For this review, take the finished solid that the model builds, in its own axes (mm). A direction names the side the tool comes from. Give positions to 0.01 mm unless a question says otherwise; leave off trailing zeros. Write each loop counter-clockwise with the first axis right and the second up, starting at its lowest first coordinate (ties: lowest second). Pieces come first, ordered by that corner, then holes.
from build123d import *

# Parameters (mm, degrees)
CHAMFER1_SIZE = 0.254
CHAMFER2_SIZE = 0.127


with BuildPart() as part:
    # Sketch1 → Revolve1 (revolve)
    with BuildSketch(Plane(origin=(0, 0, 0), x_dir=(0, 0, -1), z_dir=(1, 0, 0)), mode=Mode.PRIVATE) as revolve1_sk:
        Polygon((0, 6.35), (25.4, 6.35), (25.4, 4.6736), (15.24, 4.6736), (15.24, 3.96875), (0, 3.96875), align=None)
    revolve(revolve1_sk.sketch.rotate(Axis((0, 0, 0), (0, 0, -1)), 90), axis=Axis((0, 0, 0), (0, 0, -1)))

    # Chamfer1
    chamfer1_edges = [part.edges().sort_by_distance(p)[0] for p in [
        (-3.96875, 0, 0),
        (-4.6736, 0, -25.4),
        (-6.35, 0, -25.4),
        (-6.35, 0, 0),
    ]]
    chamfer(chamfer1_edges, length=CHAMFER1_SIZE)

    # Chamfer2
    chamfer2_edges = [part.edges().sort_by_distance(p)[0] for p in [
        (-3.96875, 0, -15.24),
    ]]
    chamfer(chamfer2_edges, length=CHAMFER2_SIZE)


solid = part.part
(1) For L1, parallel to Y at x = 0, z = -7.5; L2, parallel to Y at x = 0.25, z = -16.25; L3, parallel to Z at x = 2.25, y = -4, list the stretches that pass through material, from the lowest coordinate up.
(2) Clearance check with flat-ended pins moving along their axes: pin 1 Ø2 at (x, y) = (1, 1) entering from -Z; pin 2 Ø2 at (x, z) = (-2.5, -8) entering from -Y; pin 3 Ø1.5 at (y, z) = (2, -16.5) entering from +X; pin 4 Ø4 at (x, z) = (3.5, -11) entering from +Y. State where each tip first meets the part, or that it passes through.
(3) We need section C-C (z = -13.25). Write out the cut boundary in (x, y), and give its area (3 significant figures).
(4) The part is to be moulded in two halves that separate along X. For faces 1 (the flat face through (1.44, -4.15, 0)), 2 (the cylindrical face through (-0.86, 3.874, -7.579)), 3 (the cylindrical face through (-5.04, 3.86, -12.87)), say which applies: +X half, -X half, draft (parallel to the pull), parting line (faces both ways), or undercut.
(5) We need section D-D (z = -20.25). Write out the cut boundary in (x, y).
(6) Tool access review of faces 4 (the cylindrical face through (4.46, -1.4, -20.12)), 5 (the flat face through (1, 5, -25.4)): name each direction out of +Z, -Z, +X, -X, +Y, -Y from which nothing blocks a thin tool from reaching the whole face with its end or side.
(7) We need section A-A (x = 0). Write out the cut boundary in (y, z).
The answers:
1. L1: y = -6.35 to -3.97, 3.97 to 6.35
1. L2: y = -6.35 to -4.67, 4.67 to 6.35
1. L3: z = -15.24 to 0
2. pin 1: passes through
2. pin 2: stops at y = -6.17
2. pin 3: stops at x = 6.23
2. pin 4: stops at y = 6.17
3. outline: circle Ø12.7 at (0, 0); hole circle Ø7.94 at (0, 0)
3. area: 77.2 mm2
4. face 1: draft
4. face 2: undercut
4. face 3: parting line
5. outline: circle Ø12.7 at (0, 0); hole circle Ø9.35 at (0, 0)
6. face 4: -Z
6. face 5: -Z, +X, -X, +Y, -Y
7. outline: (-6.35, -25.15) - (-6.1, -25.4) - (-4.93, -25.4) - (-4.67, -25.15) - (-4.67, -15.24) - (-4.1, -15.24) - (-3.97, -15.11) - (-3.97, -0.25) - (-4.22, 0) - (-6.1, 0) - (-6.35, -0.25) - close; (3.97, -15.11) - (4.1, -15.24) - (4.67, -15.24) - (4.67, -25.15) - (4.93, -25.4) - (6.1, -25.4) - (6.35, -25.15) - (6.35, -0.25) - (6.1, 0) - (4.22, 0) - (3.97, -0.25) - close
